For this review, use the dimensioned drawing (mm, ordinates from the lowest corner) and the shaded views. A direction names the side the tool comes from. Coordinates: 2 decimals unless noted, no trailing zeros. Order: outer loops, then holes, each group sorted by start corner. A loop starts at its lowest first (then second) coordinate and runs counter-clockwise, first axis right, second up. Notation, with made-up numbers: (-4.75, -14.5) -> (44.25, -14.5) arc R18 cw to (44.25, 4.5) -> close; hole circle Ø4 at (-12, 62.5). An arc over 180 degrees is marked (long way). Return JSON: item names as keys, results as strings. Group by question number.
Item 1: Take a section at A-A (x = 31). Write out the cut boundary in (y, z) (1 decimal).
Item 2: Take a section at D-D (y = 20). Count the separate pieces of the cut face and the enclosed holes in it, then the cut area to 3 significant figures.
Item 3: Take a section at B-B (x = 46.5). Write out the cut boundary in (y, z) (1 decimal), then the cut area to 3 significant figures.
Item 4: For line 1 along Z through (x, y) = (31, 1.65) (1 decimal); line 2 along X through (y, z) = (11.5, 26.5); line 3 along Y through (x, z) = (16, 11) (1 decimal), list the stretches that pass through material, from the lowest coordinate up.
Item 5: Insertion check: pin 1 (19 mm diameter, centred on y = 13, z = 19, fed in from +X); pin 2 (4 mm diameter, centred on x = 3, y = 12, fed in from -Z). Each pin has a flat end and moves straight along its axis. Give the tip position at first contact, or say it passes through.
Item 6: Machinability: for the marked faces 1, 2, 3, 4 and 5, which of the approach directions +Z, -Z, +X, -X, +Y, -Y give a long, thin tool a straight path to every point of the face, cutting with its end or side? Answer none if there is none.
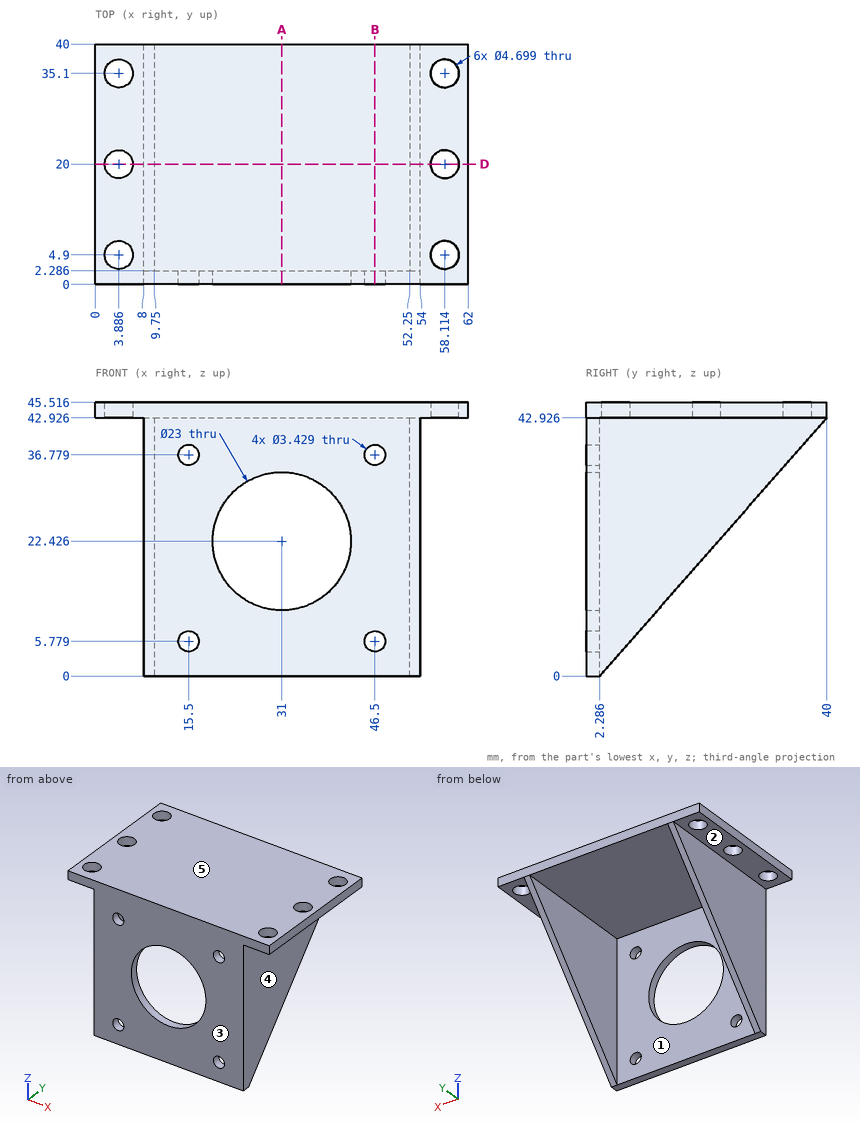
Findings below:
{
 "1": {"outline": "(0, 0) -> (2.3, 0) -> (2.3, 10.9) -> (0, 10.9) -> close; (0, 33.9) -> (2.3, 33.9) -> (2.3, 42.9) -> (40, 42.9) -> (40, 45.5) -> (0, 45.5) -> close"},
 "2": {"separate pieces": "3", "enclosed holes": "0", "area": "216 mm2"},
 "3": {"outline": "(0, 0) -> (2.3, 0) -> (2.3, 4.1) -> (0, 4.1) -> close; (0, 7.5) -> (2.3, 7.5) -> (2.3, 35.1) -> (0, 35.1) -> close; (0, 38.5) -> (2.3, 38.5) -> (2.3, 42.9) -> (40, 42.9) -> (40, 45.5) -> (0, 45.5) -> close", "area": "186 mm2"},
 "4": {"line 1": "z = 0 to 10.9, 33.9 to 45.5", "line 2": "x = 8 to 9.75, 52.25 to 54", "line 3": "y = 0 to 2.3"},
 "5": {"pin 1": "stops at x = 54", "pin 2": "stops at z = 42.93"},
 "6": {"face 1": "-Z, +Y", "face 2": "-Z, -X, +Y, -Y", "face 3": "+Z, -Z, +X, -X, -Y", "face 4": "-Z, +X, +Y, -Y", "face 5": "+Z, +X, -X, +Y, -Y"}
}
